CAD build for the part. Positions are in the model's coordinates, mm. Face numbers are marked on the shaded views. A direction names the side the tool comes from. Round coordinates to 2 decimals unless told otherwise and drop trailing zeros. Loops run counter-clockwise (first coordinate to the right, second up) from the corner with the lowest first, then second, coordinate; pieces in that order, holes last. Notation, with made-up numbers: M 48.5,43 L 83.5,43 A18 ccw 83.5,55 Z; hole C -0.75,84 d4. An arc over 180 degrees is marked long. One line per item, written item: value. Start each with the question number.
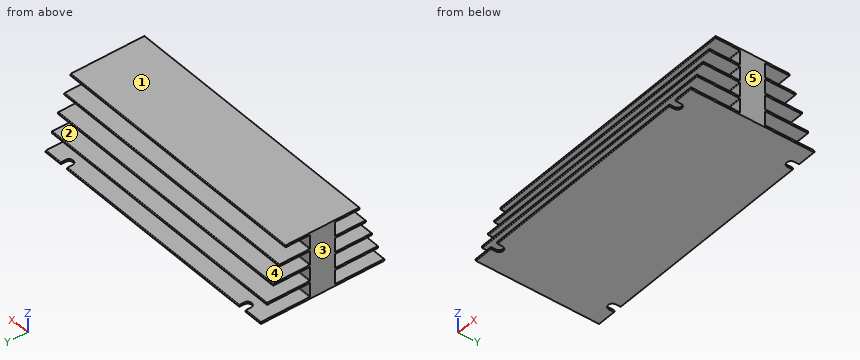
from build123d import *

# Parameters (mm, degrees)
F0_W     = 260
F0_H     = 24
F1_DEPTH = 65
F2_DEPTH = 2
F3_W     = 12
F3_H     = 2
F3_W_2   = 6
F3_W_3   = 18
F4_DEPTH = 260
F3_W_4   = 24
F3_H_2   = 13.75
F5_DEPTH = 260
F6_R     = 0.5
F7_W     = 8
F7_H     = 0.5
F7_H_2   = 4.5
F8_DEPTH = 2


# Not quite as in the source:
# - a feature names something its author has since deleted; it is built from what else it names


with BuildPart() as f1:
    # F0 (on Top) → F1 (new body)
    with BuildSketch(Plane.XY):
        with Locations((0, -24)):
            Rectangle(F0_W, F0_H)
        Rectangle(F0_W, F0_H)
        with Locations((0, 24)):
            Rectangle(F0_W, F0_H)
    extrude(amount=F1_DEPTH)

    # F0 (on Top) → F2 (join)
    with BuildSketch(Plane.XY):
        with Locations((0, -48)):
            Rectangle(F0_W, F0_H)
        with Locations((0, 48)):
            Rectangle(F0_W, F0_H)
    extrude(amount=F2_DEPTH)

    # F3 (on face) → F4 (join)
    with BuildSketch(Plane(origin=(-130, 0, 0), x_dir=(0, -1, 0), z_dir=(-1, 0, 0))):
        Polygon((36, 65), (0, 65), (0, 0), (60, 0), (60, 2), (36, 2), (12, 2), (12, 15.75), (36, 15.75), (36, 17.75), (12, 17.75), (12, 31.5), (36, 31.5), (36, 33.5), (12, 33.5), (12, 47.25), (36, 47.25), (36, 49.25), (12, 49.25), (12, 63), (36, 63), align=None)
        Polygon((0, 65), (-36, 65), (-36, 63), (-12, 63), (-12, 49.25), (-36, 49.25), (-36, 47.25), (-12, 47.25), (-12, 33.5), (-36, 33.5), (-36, 31.5), (-12, 31.5), (-12, 17.75), (-36, 17.75), (-36, 15.75), (-12, 15.75), (-12, 2), (-36, 2), (-60, 2), (-60, 0), (0, 0), align=None)
        with Locations((-42, 32.5)):
            Rectangle(F3_W, F3_H)
        with Locations((-39, 48.25)):
            Rectangle(F3_W_2, F3_H)
        with Locations((-45, 16.75)):
            Rectangle(F3_W_3, F3_H)
        with Locations((45, 16.75)):
            Rectangle(F3_W_3, F3_H)
        with Locations((42, 32.5)):
            Rectangle(F3_W, F3_H)
        with Locations((39, 48.25)):
            Rectangle(F3_W_2, F3_H)
    extrude(amount=-F4_DEPTH)

    # F3 (on face) → F5 (cut)
    with BuildSketch(Plane(origin=(-130, 0, 0), x_dir=(0, -1, 0), z_dir=(-1, 0, 0))):
        with Locations((-24, 8.875)):
            Rectangle(F3_W_4, F3_H_2)
        with Locations((-24, 56.125)):
            Rectangle(F3_W_4, F3_H_2)
        with Locations((-24, 40.375)):
            Rectangle(F3_W_4, F3_H_2)
        with Locations((-24, 24.625)):
            Rectangle(F3_W_4, F3_H_2)
        with Locations((24, 8.875)):
            Rectangle(F3_W_4, F3_H_2)
        with Locations((24, 24.625)):
            Rectangle(F3_W_4, F3_H_2)
        with Locations((24, 40.375)):
            Rectangle(F3_W_4, F3_H_2)
        with Locations((24, 56.125)):
            Rectangle(F3_W_4, F3_H_2)
    extrude(amount=-F5_DEPTH, mode=Mode.SUBTRACT)

    # F6
    f6_edges = [f1.edges().sort_by_distance(p)[0] for p in [
        (0, 36, 65),
        (0, 36, 63),
        (0, 48, 33.5),
        (0, 48, 31.5),
        (0, 54, 17.75),
        (0, 54, 15.75),
        (0, 60, 0),
        (0, 60, 2),
        (0, -60, 2),
        (0, -54, 17.75),
        (0, -48, 33.5),
        (0, -42, 49.25),
        (0, -36, 65),
        (0, -60, 0),
        (0, -54, 15.75),
        (0, -48, 31.5),
        (0, -42, 47.25),
        (0, -36, 63),
        (0, 12, 63),
        (0, 12, 49.25),
        (0, 12, 33.5),
        (0, 12, 47.25),
        (0, 12, 31.5),
        (0, 12, 15.75),
        (0, 12, 2),
        (0, -12, 63),
        (0, -12, 47.25),
        (0, -12, 31.5),
        (0, -12, 49.25),
        (0, -12, 33.5),
        (0, -12, 15.75),
        (0, -12, 17.75),
        (0, 42, 49.25),
        (0, 12, 17.75),
        (0, -12, 2),
        (0, 42, 47.25),
    ]]
    fillet(f6_edges, radius=F6_R)

    # F7 (on face) → F8 (cut)
    with BuildSketch(Plane(origin=(0, 0, 0), x_dir=(1, 0, 0), z_dir=(0, 0, -1))):
        with Locations((-108, -59.75)):
            Rectangle(F7_W, F7_H)
        with Locations((-108, -57.25)):
            Rectangle(F7_W, F7_H_2)
        with BuildLine():
            ThreePointArc((-104, -55), (-108, -51), (-112, -55))
            Line((-112, -55), (-104, -55))
        make_face()
        with Locations((-108, 59.75)):
            Rectangle(F7_W, F7_H)
        with BuildLine():
            Line((-104, 55), (-112, 55))
            ThreePointArc((-112, 55), (-108, 51), (-104, 55))
        make_face()
        with Locations((108, -59.75)):
            Rectangle(F7_W, F7_H)
        with Locations((108, -57.25)):
            Rectangle(F7_W, F7_H_2)
        with BuildLine():
            ThreePointArc((112, -55), (108, -51), (104, -55))
            Line((104, -55), (112, -55))
        make_face()
        with BuildLine():
            Line((112, 55), (104, 55))
            ThreePointArc((104, 55), (108, 51), (112, 55))
        make_face()
        with Locations((108, 59.75)):
            Rectangle(F7_W, F7_H)
        with Locations((108, 57.25)):
            Rectangle(F7_W, F7_H_2)
        with Locations((-108, 57.25)):
            Rectangle(F7_W, F7_H_2)
    extrude(amount=-F8_DEPTH, mode=Mode.SUBTRACT)


solid = f1.part
(1) Mould opens along Z. For the marked faces 1, 2 and 3 say: pulls with the +Z half, pulls with the -Z half, needs draft (parallel to the pull), parting line crosses it, or undercut.
(2) Flat gauge pins, fed straight in: P1, Ø4, axis at x = 43, z = 55, coming from the -Y side; P2, Ø4, axis at x = 4, z = 7.5, coming from the +Y side; P3, Ø14, axis at x = 57, z = 42.5, coming from the -Y side. Where does each tip first touch, or does it go through?
(3) Slice it at B-B, the plane z = 27.5. List the corners of the cut face in (x, y), and give its area (3 significant figures).
(4) Slice it at A-A, the plane y = -15.5. List the corners of the cut face in (x, z), and give its area (3 significant figures).
(5) Probe L1, parallel to Z at x = -77, y = -43; L2, parallel to Z at x = 107, y = 18; L3, parallel to Z at x = -88.5, y = -50.5. List the from-to ranges inside material, lowest first.
(6) Which spindle directions (+Z, -Z, +X, -X, +Y, -Y) get a long thin tool onto all of the face, cutting with end or side? Do the marked faces 4 and 5. Say none if no direction does.
Check result:
1. face 1: pulls with the +Z half
1. face 2: undercut
1. face 3: needs draft
2. P1: stops at y = -12
2. P2: stops at y = 12
2. P3: stops at y = -42
3. outline: M -130,-12 L 130,-12 L 130,12 L -130,12 Z
3. area: 6,240 mm^2
4. outline: M -130,0 L 130,0 L 130,2 L -130,2 Z; M -130,15.75 L 130,15.75 L 130,17.75 L -130,17.75 Z; M -130,31.5 L 130,31.5 L 130,33.5 L -130,33.5 Z; M -130,47.25 L 130,47.25 L 130,49.25 L -130,49.25 Z; M -130,63 L 130,63 L 130,65 L -130,65 Z
4. area: 2,600 mm^2
5. L1: z = 0 to 2, 15.75 to 17.75, 31.5 to 33.5
5. L2: z = 0 to 2, 15.75 to 17.75, 31.5 to 33.5, 47.25 to 49.25, 63 to 65
5. L3: z = 0 to 2, 15.75 to 17.75
6. face 4: +X, -X, +Y
6. face 5: +Z, -Z, +X, +Y, -Y
